```python
from build123d import *

# Parameters (mm, degrees)
EXTRUDE_1_DEPTH = 8
FILLET_1_R      = 0.2


with BuildPart() as part:
    # Эскиз1 → Бобышка-Вытянуть1 (new body, symmetric)
    with BuildSketch(Plane.XY):
        Polygon((4, 0), (-4, 0), (-4, -1.8), (-8, -1.8), (-8, -3.6), (-4, -6), (4, -6), (8, -3.6), (8, -1.8), (4, -1.8), align=None)
    extrude(amount=EXTRUDE_1_DEPTH, both=True)

    # Эскиз4 → Отверстие обработанное метчиком M42 (revolve, cut)
    with BuildSketch(Plane(origin=(0, 0, 0), x_dir=(0, 0, 1), z_dir=(1, 0, 0))):
        Polygon((0, 0), (0, 6), (2.15, 6), (1.65, 5.5), (1.65, 0.5), (2.15, 0), align=None)
    revolve(axis=Axis((0, 6.35, 0), (0, -1, 0)), mode=Mode.SUBTRACT)

    # Скругление1
    fillet_1_edges = [part.edges().sort_by_distance(p)[0] for p in [
        (-4, 0, 0),
        (4, 0, 0),
        (4, -1.8, 0),
        (8, -1.8, 0),
        (4, -6, 0),
        (-4, -6, 0),
        (-8, -1.8, 0),
        (-4, -1.8, 0),
    ]]
    fillet(fillet_1_edges, radius=FILLET_1_R)


solid = part.part
```
Geometry check sheet. Reference: the model listing, model coordinates, mm. A direction names the side the tool comes from. Round coordinates to 2 decimals unless told otherwise and drop trailing zeros. Loops run counter-clockwise (first coordinate to the right, second up) from the corner with the lowest first, then second, coordinate; pieces in that order, holes last. Notation, with made-up numbers: M 2.25,-9 L 42.25,-9 A15 cw 42.25,5 Z; hole C 3.5,42.5 d5. An arc over 180 degrees is marked long. Return JSON: item names as keys, results as strings. Group by question number.
(1) Scan lines: line 1 along Z through (x, y) = (0, -4.15); line 2 along X through (y, z) = (-1.55, 0); line 3 along X through (y, z) = (-2.45, -1.25). Record each from-to range of solid material in increasing order. Write a range as [from, to].
(2) Set-up check for faces 1 (the face through (-4, -1, 0)), 2 (the face through (4, -1, 0)), 3 (the face through (2, 0, 2)): record each of +Z, -Z, +X, -X, +Y, -Y from which the full face is reachable in a straight line by a thin tool's end or side.
(3) Section check A-A, the plane z = 0. Enter the section's corners in (x, y), and give its area (3 significant figures).
(4) Section check B-B, the plane y = -2.4. Enter the section's corners in (x, z).
(5) Go/stop test with flat-tipped pins: pin 1 (5 mm diameter, centred on x = -4.5, z = -1.5, fed in from +Y); pin 2 (4 mm diameter, centred on x = 0, z = 0, fed in from -Y); pin 3 (1.1 mm diameter, centred on x = -6, z = 0.5, fed in from +Y); pin 4 (1.1 mm diameter, centred on y = -1, z = 2, fed in from -X). Record where each tip stops, or that it passes through.
(6) Mould release check, pull along X, two halves, no side actions. Record for faces 4 (the face through (-1.115, -2.965, -1.216)), 5 (the face through (-8, -3, 0)), 6 (the face through (-6, -1.8, 0)): pulls with the +X half, pulls with the -X half, needs draft (parallel to the pull), parting line crosses it, or undercut.
(7) Section check D-D, the plane z = 5.75. Enter the section's corners in (x, y).
(8) Section check C-C, the plane x = 0. Enter the section's corners in (y, z).
Data:
{
 "1": {"line 1": "[-8, -1.65], [1.65, 8]", "line 2": "[-4, -1.65], [1.65, 4]", "line 3": "[-8, -1.08], [1.08, 8]"},
 "2": {"face 1": "+Z, -Z, -X, +Y", "face 2": "+Z, -Z, +X, +Y", "face 3": "+Z, -Z, +X, -X, +Y"},
 "3": {"outline": "M -8,-3.6 L -4.05,-5.97 A0.2 ccw -3.94,-6 L -2.15,-6 L -1.65,-5.5 L -1.65,-0.5 L -2.15,0 L -3.8,0 A0.2 ccw -4,-0.2 L -4,-1.6 A0.2 cw -4.2,-1.8 L -7.8,-1.8 A0.2 ccw -8,-2 Z; M 1.65,-5.5 L 2.15,-6 L 3.94,-6 A0.2 ccw 4.05,-5.97 L 8,-3.6 L 8,-2 A0.2 ccw 7.8,-1.8 L 4.2,-1.8 A0.2 cw 4,-1.6 L 4,-0.2 A0.2 ccw 3.8,0 L 2.15,0 L 1.65,-0.5 Z", "area": "51.7 mm²"},
 "4": {"outline": "M -8,-8 L 8,-8 L 8,8 L -8,8 Z; hole C 0,0 d3.3"},
 "5": {"pin 1": "y = 0", "pin 2": "y = -5.85", "pin 3": "y = -1.8", "pin 4": "x = -4"},
 "6": {"face 4": "undercut", "face 5": "pulls with the -X half", "face 6": "needs draft"},
 "7": {"outline": "M -8,-3.6 L -4.05,-5.97 A0.2 ccw -3.94,-6 L 3.94,-6 A0.2 ccw 4.05,-5.97 L 8,-3.6 L 8,-2 A0.2 ccw 7.8,-1.8 L 4.2,-1.8 A0.2 cw 4,-1.6 L 4,-0.2 A0.2 ccw 3.8,0 L -3.8,0 A0.2 ccw -4,-0.2 L -4,-1.6 A0.2 cw -4.2,-1.8 L -7.8,-1.8 A0.2 ccw -8,-2 Z"},
 "8": {"outline": "M -6,-8 L 0,-8 L 0,-2.15 L -0.5,-1.65 L -5.5,-1.65 L -6,-2.15 Z; M -6,2.15 L -5.5,1.65 L -0.5,1.65 L 0,2.15 L 0,8 L -6,8 Z"}
}
